Build history of the part. All positions in model axes, mm. A direction names the side the tool comes from. Give positions to 0.01 mm unless a question says otherwise; leave off trailing zeros. Order: outer loops, then holes, each group sorted by start corner. A loop starts at its lowest first (then second) coordinate and runs counter-clockwise, first axis right, second up. Notation, with made-up numbers: (-9.75, -29.75) - (17.25, -29.75) arc R21 ccw to (17.25, -10.75) - close; hole circle Ø2 at (-34, 77.25). An arc over 180 degrees is marked (long way). Write each question's results on one line, items separated by ' | '. Start each with the question number.
1) Tool access for faces 4 (the face through (19.5, 36, 1)), 5 (the face through (-41.5, -7, 1)), 6 (the face through (-41.5, 36, 1)): list every direction of +Z, -Z, +X, -X, +Y, -Y with a clear straight run to the whole face (end or side of a thin tool).
2) Cut at B-B on x = -37.5. List the corners of the cut face in (y, z).
3) Cut at D-D on x = 0. List the corners of the cut face in (y, z).
4) Cut at A-A on y = 41. List the corners of the cut face in (x, z).
5) Cut at C-C on z = 1. State how many separate pieces and enclosed holes the cut face has, plus the area to 3 significant figures.
6) Drill centre lines: line 1 along Y through (x, z) = (-42.5, 0.9); line 2 along X through (y, z) = (41.5, 0.25); line 3 along X through (y, z) = (-3, 1.2). Where is each one in solid material? Low to high. Write a range as from..to.
7) Two-plate mould, pull along Y, no slides. Class faces 1 (the face through (-1.27, -0.97, 0.99)), 2 (the face through (-11, 14, 0)), 3 (the face through (-40, -17, 1)): +Y half, -Y half, draft (parallel to the pull), parting line (faces both ways), or undercut.
8) Drop flat-ended pins along their axis: pin 1 Ø1 at (y, z) = (-10, 1) entering from +X; pin 2 Ø2.5 at (x, y) = (15.5, 41) entering from -Z. Give the stop position or say it passes through.
from build123d import *

# Parameters (mm, degrees)
SKETCH_1_W      = 38
SKETCH_1_H      = 54
SKETCH_1_R      = 1.6
EXTRUDE_1_DEPTH = 2
SKETCH_4_R      = 1.6
EXTRUDE_2_DEPTH = 2
CHAMFER_1_SIZE  = 2.5


with BuildPart() as part:
    # 草图1 → 凸台-拉伸1 (new body)
    with BuildSketch(Plane.XY):
        with Locations((-11, 14)):
            Rectangle(SKETCH_1_W, SKETCH_1_H)
        Circle(SKETCH_1_R, mode=Mode.SUBTRACT)
        with Locations((-7, 38.6)):
            Circle(SKETCH_1_R, mode=Mode.SUBTRACT)
    extrude(amount=EXTRUDE_1_DEPTH)

    # 草图4 → 凸台-拉伸2 (add)
    with BuildSketch(Plane.XY):
        Polygon((-33.880035193, 46), (19.5, 46), (19.5, 25), (24.5, 25), (24.5, 3), (19.5, 3), (19.5, -18), (-41.5, -18), (-41.5, 2.119651453), (-41.5, 3), (-46.5, 3), (-46.5, 25.960072655), (-41.5, 25.960072655), (-41.5, 46), align=None)
        with Locations((-37.5, 41)):
            Circle(SKETCH_4_R, mode=Mode.SUBTRACT)
        with Locations((15.5, -13)):
            Circle(SKETCH_4_R, mode=Mode.SUBTRACT)
        with Locations((-37.5, -13)):
            Circle(SKETCH_4_R, mode=Mode.SUBTRACT)
        with Locations((15.5, 41)):
            Circle(SKETCH_4_R, mode=Mode.SUBTRACT)
        with Locations((-42.5, 21)):
            Circle(SKETCH_4_R, mode=Mode.SUBTRACT)
        with Locations((20.5, 7)):
            Circle(SKETCH_4_R, mode=Mode.SUBTRACT)
        with Locations((-42.5, 7)):
            Circle(SKETCH_4_R, mode=Mode.SUBTRACT)
        with Locations((20.5, 21)):
            Circle(SKETCH_4_R, mode=Mode.SUBTRACT)
        with Locations((-7, 38.6)):
            Circle(SKETCH_4_R, mode=Mode.SUBTRACT)
        Circle(SKETCH_4_R, mode=Mode.SUBTRACT)
    extrude(amount=EXTRUDE_2_DEPTH)

    # Chamfer 1
    chamfer_1_edges = [part.edges().sort_by_distance(p)[0] for p in [
        (19.5, -18, 1),
        (19.5, 3, 1),
        (24.5, 3, 1),
        (24.5, 25, 1),
        (19.5, 25, 1),
        (19.5, 46, 1),
        (-41.5, -18, 1),
        (-41.5, 3, 1),
        (-46.5, 3, 1),
        (-41.5, 25.960072655, 1),
        (-46.5, 25.960072655, 1),
        (-41.5, 46, 1),
    ]]
    chamfer(chamfer_1_edges, length=CHAMFER_1_SIZE - 0.0001)  # a hair under: the kernel refuses the full size


solid = part.part
Results:
1) face 4: +Z, -Z, +X, +Y | face 5: +Z, -Z, -X, -Y | face 6: +Z, -Z, -X, +Y
2) outline: (-18, 0) - (-14.6, 0) - (-14.6, 2) - (-18, 2) - close; (-11.4, 0) - (39.4, 0) - (39.4, 2) - (-11.4, 2) - close; (42.6, 0) - (46, 0) - (46, 2) - (42.6, 2) - close
3) outline: (-18, 0) - (-1.6, 0) - (-1.6, 2) - (-18, 2) - close; (1.6, 0) - (46, 0) - (46, 2) - (1.6, 2) - close
4) outline: (-41.5, 0) - (-39.1, 0) - (-39.1, 2) - (-41.5, 2) - close; (-35.9, 0) - (13.9, 0) - (13.9, 2) - (-35.9, 2) - close; (17.1, 0) - (19.5, 0) - (19.5, 2) - (17.1, 2) - close
5) separate pieces: 1 | enclosed holes: 10 | area: 4,040 mm^2
6) line 1: 1.5..5.4, 8.6..19.4, 22.6..27.46 | line 2: -41.5..-39.02, -35.98..13.98, 17.02..19.5 | line 3: -41.5..19.5
7) face 1: undercut | face 2: draft | face 3: -Y half
8) pin 1: x = 19.5 | pin 2: through
